Part model, mm, in its own coordinate system. Face numbers are marked on the shaded views. Coordinates: 2 decimals unless noted, no trailing zeros. Write each loop counter-clockwise with the first axis right and the second up, starting at its lowest first coordinate (ties: lowest second). Pieces come first, ordered by that corner, then holes. Notation, with made-up numbers: (15.5, 0.25) -> (46.5, 0.25) arc R28 cw to (46.5, 29.25) -> close; hole circle Ø2 at (-34.5, 42.5). An arc over 180 degrees is marked (long way). Write item = value, one per line.
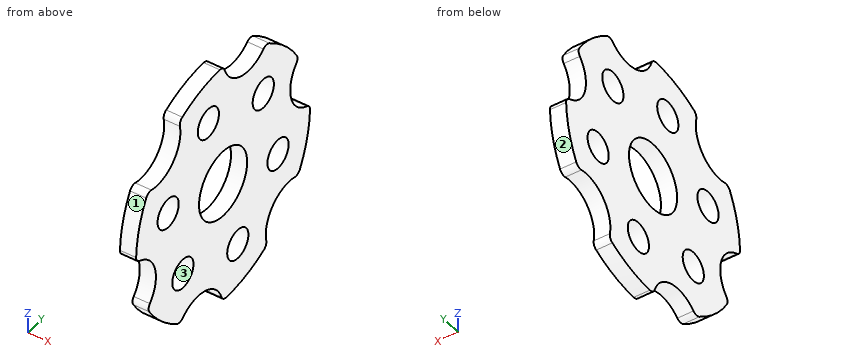
Autodesk Inventor part; units mm, degrees
ref_plane "YZ Plane" through (0, 0, 0) normal (1, 0, 0) x (0, 1, 0)
ref_plane "XZ Plane" through (0, 0, 0) normal (0, 1, 0) x (-1, 0, 0)
ref_plane "XY Plane" through (0, 0, 0) normal (0, 0, 1) x (1, 0, 0)
sketch "Sketch1" plane through (0, 0, 0) normal (1, 0, 0) x (0, 1, 0)
  circle A0 centre (0, 0) radius 57.3659
  circle A1 centre (0, 0) radius 37.4904
  circle A2 centre (26.5097, 26.5097) radius 6.985
  line L0 (0, 0) -> (26.5097, 26.5097)
  line L1 (0, 0) -> (37.4904, 0) construction
  circle A3 centre (-9.7032, 36.2129) radius 6.985
  circle A4 centre (-36.2129, 9.7032) radius 6.985
  circle A5 centre (-26.5097, -26.5097) radius 6.985
  circle A6 centre (9.7032, -36.2129) radius 6.985
  circle A7 centre (36.2129, -9.7032) radius 6.985
  circle A8 centre (0, 0) radius 15.875
  circle A9 centre (60.1365, 16.1135) radius 15.875
  line L2 (0, 0) -> (62.2818, 0) construction
  line L3 (0, 0) -> (54.4204, 0) construction
  line L4 (0, 0) -> (47.0027, 0) construction
  line L5 (0, 0) -> (74.4134, 19.939)
  line L6 (0, 0) -> (77.0384, 0) construction
  circle A10 centre (0, 0) radius 15.875
  circle A11 centre (16.1135, 60.1365) radius 15.875
  circle A12 centre (0, 0) radius 15.875
  circle A13 centre (-44.023, 44.023) radius 15.875
  circle A14 centre (0, 0) radius 15.875
  circle A15 centre (-60.1365, -16.1135) radius 15.875
  circle A16 centre (0, 0) radius 15.875
  circle A17 centre (-16.1135, -60.1365) radius 15.875
  circle A18 centre (0, 0) radius 15.875
  circle A19 centre (44.023, -44.023) radius 15.875
  point P0 (36.2129, 9.7032)
  point P1 (49.9198, 28.264)
  point P2 (28.264, 49.9198)
  point P3 (0.4825, 57.3639)
  point P4 (-29.0998, 49.4373)
  point P5 (-49.4373, 29.0998)
  point P6 (-57.3639, -0.4825)
  point P7 (-49.9198, -28.264)
  point P8 (-28.264, -49.9198)
  point P9 (-0.4825, -57.3639)
  point P10 (29.0998, -49.4373)
  point P11 (49.4373, -29.0998)
  point P12 (57.3639, 0.4825)
  dimension "d0" = 114.7318
  dimension "d1" = 74.9808
  dimension "d2" = 13.97
  dimension "d3" = 45
  dimension "d6" = 360
  dimension "d8" = 31.75
  dimension "d12" = 31.75
  dimension "d16" = 15
  dimension "d19" = 360
extrude "Extrusion1" add sketch "Sketch1" along normal blind 7.5184 contours A1 A7 A6 A5 A4 A3 A2 L0 A8 L5 | L5 A8 L0 A2 A1 | A0 A19 A17 A15 A13 A11 A9
fillet "Fillet1" radius 3.175 12 edges at (3.7592, 57.3639, 0.4825) (3.7592, 49.9198, 28.264) (3.7592, 29.0998, -49.4373) (3.7592, 49.4373, -29.0998) (3.7592, -0.4825, -57.3639) (3.7592, -28.264, -49.9198) (3.7592, -49.9198, -28.264) (3.7592, -57.3639, -0.4825) (3.7592, -49.4373, 29.0998) (3.7592, -29.0998, 49.4373) (3.7592, 0.4825, 57.3639) (3.7592, 28.264, 49.9198)
properties part number "Flex_Giubo_V1"
Q1. Saw through at D-D on x = 4. Count the separate pieces of the cut face and the enclosed holes in it, and give its area (3 significant figures).
Model answer:
separate_pieces = 1
enclosed_holes = 7
area = 7,270 mm²
Q2. Probe line 1 (Y direction, x = 7, z = -30); line 2 (Y direction, x = 5.5, z = -8.5); line 3 (Z direction, x = 4.5, y = -45.5). List the from-to ranges inside material, lowest first. Write a range as from..to.
Model answer:
line_1 = -48.85..-32.56, -20.46..6.51, 12.9..36.58
line_2 = -46.21..-13.41, 13.41..29.33, 43.09..56.73
line_3 = -34.94..-22.26, -9.97..28.22
Q3. Saw through at C-C on y = -18. Give the cut face in (x, z).
Model answer:
outline = (0, -44.37) -> (7.52, -44.37) -> (7.52, 54.47) -> (0, 54.47) -> close
Q4. Pin check, flat tips, straight feed: pin 1 (1.5 mm diameter, centred on x = 1.5, y = -6.5, fed in from +Z); pin 2 (1.5 mm diameter, centred on x = 5, y = -44.5, fed in from +Z); pin 3 (2 mm diameter, centred on x = 4.5, y = -17, fed in from -Z). Stop position of each tip, or through.
Model answer:
pin_1 = 57.08
pin_2 = 28.2
pin_3 = -44.37
Q5. Mould opens along Z. For the marked faces 1, 2 and 3 say: released by +Z, released by -Z, zero draft, split by the parting line, or undercut.
Model answer:
face_1 = released by +Z
face_2 = released by -Z
face_3 = undercut
Q6. Saw through at B-B on z = -25. Give the cut face in (x, y).
Model answer:
outline = (0, -46.98) -> (7.52, -46.98) -> (7.52, -33.33) -> (0, -33.33) -> close; (0, -19.69) -> (7.52, -19.69) -> (7.52, 51.63) -> (0, 51.63) -> close
Q7. Saw through at A-A on z = 38.5. Give the cut face in (x, y).
Model answer:
outline = (0, -29.14) -> (7.52, -29.14) -> (7.52, -16.3) -> (0, -16.3) -> close; (0, -3.1) -> (7.52, -3.1) -> (7.52, 42.53) -> (0, 42.53) -> close
